Part model, mm, in its own coordinate system. A direction names the side the tool comes from. Give positions to 0.01 mm unless a question says otherwise; leave off trailing zeros. Write each loop counter-clockwise with the first axis right and the second up, starting at its lowest first coordinate (ties: lowest second). Pieces come first, ordered by that corner, then holes. Notation, with made-up numbers: M -1,0.25 L 42,0.25 A18 cw 42,8.25 Z; hole C 44.25,18 d3. An arc over 180 degrees is marked long. Use CSV: the item, a comma, the result in double quotes. Start each with the question number.
1. Band-saw the part on D-D, the plane z = -3.5. List the corners of the cut face in (x, y).
2. Band-saw the part on A-A, the plane x = -30.8. List the corners of the cut face in (y, z).
3. 3-axis set-ups, long thin cutter, end or side, ignore diameter. For faces 1 (the face through (-35, 1, -16)), 2 (the face through (36, 1, 12.4)), 3 (the face through (36, 1, 5.6)), 4 (the face through (-35, 1, -1)): which of +Z, -Z, +X, -X, +Y, -Y reach the whole face in a straight line?
4. Drop flat-ended pins along their axis: pin 1 Ø0.6 at (x, y) = (36.5, 1) entering from +Z; pin 2 Ø4 at (x, z) = (-22.5, -11) entering from -Y; pin 3 Ø0.8 at (x, y) = (21.5, 1) entering from -Z; pin 4 Ø1.2 at (y, z) = (1.5, -3) entering from -X. Give the stop position or say it passes through.
5. Drill centre lines: line 1 along X through (y, z) = (1.7, -14.5); line 2 along X through (y, z) = (1.45, 11); line 3 along Z through (x, y) = (-30.8, 1). Where is each one in solid material? Low to high. Write a range as from..to.
6. Band-saw the part on C-C, the plane y = 1.6. Count the separate pieces of the cut face and the enclosed holes in it, then the cut area to 3 significant figures.
7. Mould opens along Z. For faces 5 (the face through (24.5, 1, 11)), 6 (the face through (0, 1, 17.5)), 7 (the face through (-10, 1, -17.5)) say: pulls with the +Z half, pulls with the -Z half, needs draft (parallel to the pull), parting line crosses it, or undercut.
8. Band-saw the part on B-B, the plane x = -19.5. List the corners of the cut face in (y, z), then the cut area to 4 significant figures.
from build123d import *

# Parameters (mm, degrees)
SKETCH_1_W          = 76
SKETCH_1_H          = 35
EXTRUDE_1_DEPTH     = 2.5
SKETCH_2_W          = 13
SKETCH_2_H          = 3.5
CUT_EXTRUDE_1_DEPTH = 3.5
SKETCH_3_W          = 3
SKETCH_3_H          = 5.1
SKETCH_3_H_2        = 3.1
SKETCH_3_H_3        = 13.2
CUT_EXTRUDE_2_DEPTH = 3.5
FILLET_1_R          = 1
SKETCH_4_R          = 1.5
SKETCH_4_W          = 9.9
SKETCH_4_H          = 4.5
CUT_EXTRUDE_3_DEPTH = 3.5


with BuildPart() as part:
    # 草图1 → 凸台-拉伸1 (new body)
    with BuildSketch(Plane(origin=(0, 0, 0), x_dir=(1, 0, 0), z_dir=(0, 1, 0))):
        Rectangle(SKETCH_1_W, SKETCH_1_H)
    extrude(amount=EXTRUDE_1_DEPTH)

    # 草图2 → 切除-拉伸1 (cut, through all)
    with BuildSketch(Plane(origin=(0, 2.5, 0), x_dir=(1, 0, 0), z_dir=(0, 1, 0))):
        with Locations((-18, -10.75)):
            Rectangle(SKETCH_2_W, SKETCH_2_H)
        with Locations((18, -10.75)):
            Rectangle(SKETCH_2_W, SKETCH_2_H)
    extrude(amount=-CUT_EXTRUDE_1_DEPTH, mode=Mode.SUBTRACT)

    # 草图3 → 切除-拉伸2 (cut, through all)
    with BuildSketch(Plane(origin=(0, 2.5, 0), x_dir=(1, 0, 0), z_dir=(0, 1, 0))):
        with Locations((-36.5, -14.95)):
            Rectangle(SKETCH_3_W, SKETCH_3_H)
        with Locations((-36.5, 15.95)):
            Rectangle(SKETCH_3_W, SKETCH_3_H_2)
        with Locations((-36.5, 1)):
            Rectangle(SKETCH_3_W, SKETCH_3_H_3)
        with Locations((36.5, -14.95)):
            Rectangle(SKETCH_3_W, SKETCH_3_H)
        with Locations((36.5, 1)):
            Rectangle(SKETCH_3_W, SKETCH_3_H_3)
        with Locations((36.5, 15.95)):
            Rectangle(SKETCH_3_W, SKETCH_3_H_2)
    extrude(amount=-CUT_EXTRUDE_2_DEPTH, mode=Mode.SUBTRACT)

    # 圆角1
    fillet_1_edges = [part.edges().sort_by_distance(p)[0] for p in [
        (38, 1.25, -7.6),
        (38, 1.25, 5.6),
        (38, 1.25, -14.4),
        (-38, 1.25, 12.4),
        (-38, 1.25, -14.4),
        (-38, 1.25, 5.6),
        (-38, 1.25, -7.6),
        (38, 1.25, 12.4),
    ]]
    fillet(fillet_1_edges, radius=FILLET_1_R)

    # 草图4 → 切除-拉伸3 (cut, through all)
    with BuildSketch(Plane(origin=(0, 2.5, 0), x_dir=(1, 0, 0), z_dir=(0, 1, 0))):
        with Locations((-30.8, 14.5)):
            Circle(SKETCH_4_R)
        with Locations((21.018135054, 15.25)):
            Rectangle(SKETCH_4_W, SKETCH_4_H)
    extrude(amount=-CUT_EXTRUDE_3_DEPTH, mode=Mode.SUBTRACT)


solid = part.part
Output:
1,outline,"M -35,0 L 35,0 L 35,2.5 L -35,2.5 Z"
2,outline,"M 0,-17.5 L 2.5,-17.5 L 2.5,-16 L 0,-16 Z; M 0,-13 L 2.5,-13 L 2.5,17.5 L 0,17.5 Z"
3,face 1,"-Z, -X, +Y, -Y"
3,face 2,"+Z, +X, +Y, -Y"
3,face 3,"+X, +Y, -Y"
3,face 4,"-X, +Y, -Y"
4,pin 1,"stops at z = 12.4"
4,pin 2,"stops at y = 0"
4,pin 3,"stops at z = -13"
4,pin 4,"stops at x = -35"
5,line 1,"x = -35..-32.3, -29.3..16.07, 25.97..35"
5,line 2,"x = -38..-24.5, -11.5..11.5, 24.5..38"
5,line 3,"z = -17.5..-16, -13..17.5"
6,separate pieces,"1"
6,enclosed holes,"3"
6,area,"2,390 mm²"
7,face 5,"undercut"
7,face 6,"pulls with the +Z half"
7,face 7,"pulls with the -Z half"
8,outline,"M 0,-17.5 L 2.5,-17.5 L 2.5,9 L 0,9 Z; M 0,12.5 L 2.5,12.5 L 2.5,17.5 L 0,17.5 Z"
8,area,"78.75 mm²"
